from build123d import *

# Parameters (mm, degrees)
ESBO_O1_W                                            = 42.10000000000001
ESBO_O1_H                                            = 42.10000000000002
RESSALTO_EXTRUS_O1_DEPTH                             = 4
ESBO_O2_R                                            = 12.000000000000007
CORTE_EXTRUS_O1_DEPTH                                = 8
ESCAREADO_PARA_PARAFUSO_DE_M_QUINA_COM_C_D           = 3.2
ESCAREADO_PARA_PARAFUSO_DE_M_QUINA_COM_C_CSINK_D     = 6.3
ESCAREADO_PARA_PARAFUSO_DE_M_QUINA_COM_C_CSINK_ANGLE = 90
RESSALTO_EXTRUS_O2_DEPTH                             = 10
ESBO_O6_R                                            = 3.5000000000000075
CORTE_EXTRUS_O2_DEPTH                                = 10.000000000000002
FURO_COM_FOLGA_DE_M31_D                              = 3.2
FILETE1_R                                            = 5
CORTE_EXTRUS_O6_DEPTH                                = 22.500000000000007
CHANFRO1_SIZE                                        = 2.7
SKETCH2_W                                            = 42.10000000000001
SKETCH2_H                                            = 14.000000000000002
SKETCH2_R                                            = 1.5999999999999908
BOSS_EXTRUDE1_DEPTH                                  = 1


with BuildPart() as part:
    # Esboço1 → Ressalto-extrusão1 (new body)
    with BuildSketch(Plane.XY):
        with Locations((87.32270610713223, -330.71568115646056)):
            Rectangle(ESBO_O1_W, ESBO_O1_H)
    extrude(amount=RESSALTO_EXTRUS_O1_DEPTH)

    # Esboço2 → Corte-extrusão1 (cut)
    with BuildSketch(Plane.XY.offset(4)):
        with Locations((87.32270610713225, -330.71568115646056)):
            Circle(ESBO_O2_R)
    extrude(amount=-CORTE_EXTRUS_O1_DEPTH, mode=Mode.SUBTRACT)

    # Escareado para parafuso de máquina com cabeça chata de M31 (through all)
    with Locations(Plane.XY.offset(4)):
        with Locations((102.822706107, -346.215681156), (102.822706107, -315.215681156), (71.822706107, -315.215681156), (71.822706107, -346.215681156)):
            CounterSinkHole(ESCAREADO_PARA_PARAFUSO_DE_M_QUINA_COM_C_D / 2, ESCAREADO_PARA_PARAFUSO_DE_M_QUINA_COM_C_CSINK_D / 2, counter_sink_angle=ESCAREADO_PARA_PARAFUSO_DE_M_QUINA_COM_C_CSINK_ANGLE)

    # Esboço5 → Ressalto-extrusão2 (add)
    with BuildSketch(Plane.XY.offset(4)):
        with BuildLine():
            Line((99.98357100649832, -333.66568115646055), (108.37270610713225, -333.66568115646055))
            Line((108.37270610713225, -333.66568115646055), (108.37270610713225, -309.66568115646055))
            Line((108.37270610713225, -309.66568115646055), (66.27270610713224, -309.66568115646055))
            Line((66.27270610713224, -309.66568115646055), (66.27270610713224, -333.66568115646055))
            Line((66.27270610713224, -333.66568115646055), (74.66184120776617, -333.66568115646055))
            ThreePointArc((74.66184120776617, -333.66568115646055), (87.32270610713225, -317.71568115646056), (99.98357100649832, -333.66568115646055))
        make_face()
    extrude(amount=RESSALTO_EXTRUS_O2_DEPTH)

    # Esboço6 → Corte-extrusão2 (cut)
    with BuildSketch(Plane.XY.offset(14)):
        with Locations((71.82270610713223, -315.21568115646056)):
            Circle(ESBO_O6_R)
        with Locations((102.82270610713226, -315.21568115646056)):
            Circle(ESBO_O6_R)
    extrude(amount=-CORTE_EXTRUS_O2_DEPTH, mode=Mode.SUBTRACT)

    # Furo com folga de M31 (through all)
    with Locations(Plane(origin=(0, -309.66568115646055, 0), x_dir=(1, 0, 0), z_dir=(0, 1, 0))):
        with Locations((103.359135837, -8.012655369), (71.286276377, -8.012655369)):
            Hole(FURO_COM_FOLGA_DE_M31_D / 2)

    # Filete1
    # the kernel refuses this fillet: 5 mm, written as the material it adds along each edge
    with BuildSketch(Plane(origin=(87.48357100649832, -333.66568115646055, 4), x_dir=(0, -1, 0), z_dir=(1, 0, 0))) as filete1_piece_1_section:
        with BuildLine():
            CenterArc((FILETE1_R, -FILETE1_R), FILETE1_R, 90, 90)
            Line((0, -FILETE1_R), (0, 0))
            Line((0, 0), (FILETE1_R, 0))
        make_face()
    filete1_piece_1 = extrude(amount=20.889135100633922, mode=Mode.PRIVATE)
    filete1_piece_1 = filete1_piece_1 - Plane(origin=(87.32270610713225, -330.71568115646056, 5.015859225762799), x_dir=(-0.9739126845666216, -0.22692307692307614, 0), z_dir=(0, 0, -1)) * Cylinder(12.999999999999995, 62, mode=Mode.PRIVATE)
    filete1_piece_1 = filete1_piece_1 - Plane(origin=(103.359135837, -334.8905504329836, 8.012655369), x_dir=(-1, 0, 0), z_dir=(0, -1, 0)) * Cylinder(1.6, 62, mode=Mode.PRIVATE)
    add(filete1_piece_1)
    with BuildSketch(Plane(origin=(66.27270610713224, -333.66568115646055, 4), x_dir=(0, -1, 0), z_dir=(1, 0, 0))) as filete1_piece_2_section:
        with BuildLine():
            CenterArc((FILETE1_R, -FILETE1_R), FILETE1_R, 90, 90)
            Line((0, -FILETE1_R), (0, 0))
            Line((0, 0), (FILETE1_R, 0))
        make_face()
    filete1_piece_2 = extrude(amount=20.889135100633936, mode=Mode.PRIVATE)
    filete1_piece_2 = filete1_piece_2 - Plane(origin=(87.32270610713225, -330.71568115646056, 5.01585849038902), x_dir=(-0.9739126845666216, -0.22692307692307614, 0), z_dir=(0, 0, -1)) * Cylinder(12.999999999999995, 62, mode=Mode.PRIVATE)
    filete1_piece_2 = filete1_piece_2 - Plane(origin=(71.286276377, -334.8905494522985, 8.012655369), x_dir=(-1, 0, 0), z_dir=(0, -1, 0)) * Cylinder(1.6, 62, mode=Mode.PRIVATE)
    add(filete1_piece_2)
    # the kernel refuses this fillet: 5 mm, written as the material it takes off along each edge
    with BuildSketch(Plane(origin=(87.32270610713225, -330.71568115646056, 14), x_dir=(-0.36935058707522056, -0.9292901289840487, 0), z_dir=(0.9292901289840487, -0.36935058707522056, 0))) as filete1_2_piece_1:
        with BuildLine():
            CenterArc((12.999999999999979 + FILETE1_R, FILETE1_R), FILETE1_R, 180, 90)
            Line((12.999999999999979 + FILETE1_R, 0), (12.999999999999979, 0))
            Line((12.999999999999979, 0), (12.999999999999984, FILETE1_R))
        make_face()
    revolve(axis=Axis((87.32270610713225, -330.71568115646056, 14), (0, 0, -1)), revolution_arc=316.648856226302, mode=Mode.SUBTRACT)
    with BuildSketch(Plane(origin=(87.48357100649832, -333.66568115646055, 14), x_dir=(0, 0, -1), z_dir=(1, 0, 0))) as filete1_2_piece_2:
        with BuildLine():
            CenterArc((FILETE1_R, FILETE1_R), FILETE1_R, 180, 90)
            Line((0, FILETE1_R), (0, 0))
            Line((0, 0), (FILETE1_R, 0))
        make_face()
    extrude(amount=33.38913510063392, mode=Mode.SUBTRACT)
    with BuildSketch(Plane(origin=(53.77270610713224, -333.66568115646055, 14), x_dir=(0, 1, 0), z_dir=(1, 0, 0))) as filete1_2_piece_3:
        with BuildLine():
            CenterArc((FILETE1_R, -FILETE1_R), FILETE1_R, 90, 90)
            Line((0, -FILETE1_R), (0, 0))
            Line((0, 0), (FILETE1_R, 0))
        make_face()
    extrude(amount=33.389135100633936, mode=Mode.SUBTRACT)

    # Esboço13 → Corte-extrusão6 (cut)
    with BuildSketch(Plane.XZ.offset(351.7656811564606)):
        Polygon((74.0362763774125, 9.60036860941331), (71.28627637741243, 11.188081849684735), (68.53627637741243, 9.600368609413174), (68.53627637741253, 6.424942128870199), (71.2862763774126, 4.837228888598795), (74.03627637741259, 6.424942128870374), align=None)
        Polygon((106.10913583685199, 9.600368609413255), (103.35913583685196, 11.188081849684727), (100.60913583685196, 9.600368609413236), (100.60913583685199, 6.424942128870286), (103.359135836852, 4.837228888598834), (106.109135836852, 6.424942128870341), align=None)
    extrude(amount=-CORTE_EXTRUS_O6_DEPTH, mode=Mode.SUBTRACT)

    # Chanfro1
    chanfro1_edges = [part.edges().sort_by_distance(p)[0] for p in [
        (66.27270610713224, -351.7656811564606, 2),
        (108.37270610713225, -351.7656811564606, 2),
    ]]
    chamfer(chanfro1_edges, length=CHANFRO1_SIZE)

    # Sketch2 → Boss-Extrude1 (add)
    with BuildSketch(Plane(origin=(0, -309.66568115646055, 0), x_dir=(1, 0, 0), z_dir=(0, 1, 0))):
        with Locations((87.32270610713223, -7.000000000000001)):
            Rectangle(SKETCH2_W, SKETCH2_H)
        with Locations(Location((71.2862763774125, -8.012655369141836, 0), (0, 0, 270))):
            Circle(SKETCH2_R, mode=Mode.SUBTRACT)
        with Locations(Location((103.35913583685199, -8.012655369141836, 0), (0, 0, 270))):
            Circle(SKETCH2_R, mode=Mode.SUBTRACT)
    extrude(amount=BOSS_EXTRUDE1_DEPTH)


solid = part.part
For this review, take the finished solid that the model builds, in its own axes (mm). A direction names the side the tool comes from. Give positions to 0.01 mm unless a question says otherwise; leave off trailing zeros. Loops run counter-clockwise (first coordinate to the right, second up) from the corner with the lowest first, then second, coordinate; pieces in that order, holes last. Notation, with made-up numbers: M -9,35 L 7,35 A32 ccw 7,70 Z; hole C 70.5,41 d3. An arc over 180 degrees is marked long. Answer as a JSON object with one key per item and string values. Group by question number.
Q1. Add section B-B on z = 1. Give the boundary of the cut face in (x, y).
Q2. Insertion check: P1, Ø4, axis at x = 71.82, y = -315.22, coming from the -Z side; P2, Ø4, axis at x = 102.82, y = -315.22, coming from the +Z side; P3, Ø4, axis at x = 81, z = 10.5, coming from the -Y side; P4, Ø2, axis at x = 73, y = -315, coming from the +Z side. Each pin has a flat end and moves straight along its axis. Give the tip position at first contact, or say it passes through.
Q3. Add section C-C on z = 10.25. Give the boundary of the cut face in (x, y), and give its area (3 significant figures).
Q4. Mouldability with a two-part tool opening along Y and no side actions: class faces 3 (the flat face through (72.64, -331.89, 5.62)), 4 (the cylindrical face through (103.17, -316.778, 1.208)), 5 (the flat face through (105, -329.266, 7)), 6 (the flat face through (87, -308.666, 7)) as +Y half, -Y half, draft (parallel to the pull), parting line (faces both ways), or undercut.
Q5. Add section D-D on y = -323. Give the number of separate pieces and of enclosed holes in the cut face, and give its area (3 significant figures).
Q6. Add section A-A on y = -335. Give the boundary of the cut face in (x, z).
Q7. Tool access review of faces 1 (the flat face through (70, -329.266, 6.6)), 2 (the cylindrical face through (72.17, -347.778, 1.208)): name each direction out of +Z, -Z, +X, -X, +Y, -Y from which nothing blocks a thin tool from reaching the whole face with its end or side.
Q8. For probe 1 along X at (y, z) = (-315, 13); probe 2 along X at (y, z) = (-312, 4.75); probe 3 along Z at (x, y) = (81.5, -349.5), list the stretches that pass through material, from the lowest coordinate up. Write a range as [from, to].
Checked values:
{
 "1": {"outline": "M 66.27,-349.07 L 68.97,-351.77 L 105.67,-351.77 L 108.37,-349.07 L 108.37,-308.67 L 66.27,-308.67 Z; hole C 71.82,-346.22 d3.2; hole C 71.82,-315.22 d3.2; hole C 87.32,-330.72 d24; hole C 102.82,-346.22 d3.2; hole C 102.82,-315.22 d3.2"},
 "2": {"P1": "z = 0", "P2": "z = 2.86", "P3": "y = -320.55", "P4": "z = 3.05"},
 "3": {"outline": "M 66.27,-333.51 L 69.66,-333.51 L 69.66,-329.27 L 72.91,-329.27 L 72.91,-333.51 L 74.46,-333.51 A13.16 cw long 100.18,-333.51 L 101.73,-333.51 L 101.73,-329.27 L 104.98,-329.27 L 104.98,-333.51 L 108.37,-333.51 L 108.37,-308.67 L 66.27,-308.67 Z; hole C 71.82,-315.22 d7; hole C 102.82,-315.22 d7", "area": "596 mm²"},
 "4": {"face 3": "draft", "face 4": "undercut", "face 5": "-Y half", "face 6": "+Y half"},
 "5": {"separate pieces": "2", "enclosed holes": "2", "area": "278 mm²"},
 "6": {"outline": "M 66.27,0 L 76.11,0 L 76.11,4 L 75.05,4 L 75.05,5.6 L 72.61,5.6 L 71.29,4.84 L 69.97,5.6 L 66.27,5.6 Z; M 98.53,0 L 108.37,0 L 108.37,5.6 L 104.68,5.6 L 103.36,4.84 L 102.04,5.6 L 99.6,5.6 L 99.6,4 L 98.53,4 Z"},
 "7": {"face 1": "-Y", "face 2": "+Z, -Z"},
 "8": {"probe 1": "[66.27, 68.33], [75.32, 99.33], [106.32, 108.37]", "probe 2": "[66.27, 70.44], [73.2, 101.44], [104.2, 108.37]", "probe 3": "[0, 4]"}
}
